CAD build for the part. Positions are in the model's coordinates, mm. A direction names the side the tool comes from. Round coordinates to 2 decimals unless told otherwise and drop trailing zeros. Loops run counter-clockwise (first coordinate to the right, second up) from the corner with the lowest first, then second, coordinate; pieces in that order, holes last.
from build123d import *

# Parameters (mm, degrees)
SKETCH_1_W          = 27.7
SKETCH_1_H          = 27.5
EXTRUDE_1_DEPTH     = 2
SKETCH_2_R          = 0.75
SKETCH_2_W          = 18
SKETCH_2_H          = 4.15
CUT_EXTRUDE_1_DEPTH = 20.61848618
SKETCH_2_3_W        = 25
SKETCH_2_3_H        = 19
CUT_EXTRUDE_2_DEPTH = 1
EXTRUDE_START       = -1
SKETCH_3_R          = 0.7
EXTRUDE_2_DEPTH     = 2


with BuildPart() as part:
    # 草图1 → 凸台-拉伸1 (new body)
    with BuildSketch(Plane.XY):
        Rectangle(SKETCH_1_W, SKETCH_1_H)
    extrude(amount=EXTRUDE_1_DEPTH)

    # 草图2 → 切除-拉伸1 (cut, through all)
    with BuildSketch(Plane.XY.offset(2)):
        with Locations((-11.7, 11.85)):
            Circle(SKETCH_2_R)
        with Locations((11.7, 11.85)):
            Circle(SKETCH_2_R)
        with Locations((-11.7, -11.85)):
            Circle(SKETCH_2_R)
        with Locations((11.7, -11.85)):
            Circle(SKETCH_2_R)
        with Locations((0, 11.675)):
            Rectangle(SKETCH_2_W, SKETCH_2_H)
    extrude(amount=-CUT_EXTRUDE_1_DEPTH, mode=Mode.SUBTRACT)

    # 草图2<3> → 切除-拉伸2 (cut)
    with BuildSketch(Plane.XY.offset(2)):
        with Locations((0, 0.1)):
            Rectangle(SKETCH_2_3_W, SKETCH_2_3_H)
    extrude(amount=-CUT_EXTRUDE_2_DEPTH, mode=Mode.SUBTRACT)

    # 草图3 → 凸台-拉伸2 (add)
    # profile 1 of 2: a face of its own
    with BuildSketch(Plane.XY.offset(1).offset(EXTRUDE_START)):
        Polygon((-17.5, -8.75), (-12.5, -8.75), (-12.5, -3.75), (-17.5, -3.75), (-17.5, -4.396520298), align=None)
        with Locations((-15.5, -5.75)):
            Circle(SKETCH_3_R, mode=Mode.SUBTRACT)
    # profile 2 of 2: a face of its own
    with BuildSketch(Plane.XY.offset(1).offset(EXTRUDE_START)):
        Polygon((12.5, -8.75), (17.5, -8.75), (17.5, -4.396520298), (17.5, -3.75), (12.5, -3.75), align=None)
        with Locations((15.5, -5.75)):
            Circle(SKETCH_3_R, mode=Mode.SUBTRACT)
    extrude(amount=EXTRUDE_2_DEPTH)


solid = part.part
Item 1: Cut at A-A (x = -15.5). List the corners of the cut face in (y, z), plus the area to 3 significant figures.
Verdict:
outline: (-8.75, 0) - (-6.45, 0) - (-6.45, 2) - (-8.75, 2) - close; (-5.05, 0) - (-3.75, 0) - (-3.75, 2) - (-5.05, 2) - close
area: 7.20 mm2
Item 2: Mould opens along Y. For faces 6 (the cylindrical face through (12.415, 12.075, 1.014)), 7 (the flat face through (0, -13.75, 1)), 8 (the flat face through (-17.5, -6, 1)) say: released by +Y, released by -Y, zero draft, split by the parting line, or undercut.
Verdict:
face 6: undercut
face 7: released by -Y
face 8: zero draft
Item 3: Cut at D-D (z = 1.55). List the corners of the cut face in (x, y), plus the area to 3 significant figures.
Verdict:
outline: (-17.5, -8.75) - (-13.85, -8.75) - (-13.85, -13.75) - (13.85, -13.75) - (13.85, -8.75) - (17.5, -8.75) - (17.5, -3.75) - (13.85, -3.75) - (13.85, 13.75) - (9, 13.75) - (9, 9.6) - (12.5, 9.6) - (12.5, -9.4) - (-12.5, -9.4) - (-12.5, 9.6) - (-9, 9.6) - (-9, 13.75) - (-13.85, 13.75) - (-13.85, -3.75) - (-17.5, -3.75) - close; hole circle Ø1.4 at (-15.5, -5.75); hole circle Ø1.5 at (-11.7, -11.85); hole circle Ø1.5 at (-11.7, 11.85); hole circle Ø1.5 at (11.7, -11.85); hole circle Ø1.5 at (11.7, 11.85); hole circle Ø1.4 at (15.5, -5.75)
area: 238 mm2
Item 4: Cut at C-C (y = 11.85). List the corners of the cut face in (x, z), plus the area to 3 significant figures.
Verdict:
outline: (-13.85, 0) - (-12.45, 0) - (-12.45, 2) - (-13.85, 2) - close; (-10.95, 0) - (-9, 0) - (-9, 2) - (-10.95, 2) - close; (9, 0) - (10.95, 0) - (10.95, 2) - (9, 2) - close; (12.45, 0) - (13.85, 0) - (13.85, 2) - (12.45, 2) - close
area: 13.4 mm2
Item 5: Wall check: L1, parallel to Y at x = 11.7, z = 0.5; L2, parallel to Y at x = -11.7, z = 1.15; L3, parallel to X at y = 9.25, z = 1.2. Give the ranges that are in metal, low to high.
Verdict:
L1: y = -13.75 to -12.6, -11.1 to 11.1, 12.6 to 13.75
L2: y = -13.75 to -12.6, -11.1 to -9.4, 9.6 to 11.1, 12.6 to 13.75
L3: x = -13.85 to -12.5, 12.5 to 13.85
Item 6: Flat gauge pins, fed straight in: P1, Ø1.1, axis at x = 3, z = 0.5, coming from the +Y side; P2, Ø1, axis at x = 15.5, z = 1, coming from the -Y side; P3, Ø1.1, axis at y = 1.5, z = 1.5, coming from the -X side. Where does each tip first touch, or does it go through?
Verdict:
P1: stops at y = 9.6
P2: stops at y = -8.75
P3: stops at x = -13.85
Item 7: Cut at B-B (y = -5.75). List the corners of the cut face in (x, z), plus the area to 3 significant figures.
Verdict:
outline: (-17.5, 0) - (-16.2, 0) - (-16.2, 2) - (-17.5, 2) - close; (-14.8, 0) - (14.8, 0) - (14.8, 2) - (12.5, 2) - (12.5, 1) - (-12.5, 1) - (-12.5, 2) - (-14.8, 2) - close; (16.2, 0) - (17.5, 0) - (17.5, 2) - (16.2, 2) - close
area: 39.4 mm2
Item 8: 3-axis set-ups, long thin cutter, end or side, ignore diameter. For faces 1 (the flat face through (-16, -3.75, 1)), 2 (the flat face through (16, -3.75, 1)), 3 (the flat face through (-0.1, 9.6, 0.5)), 4 (the flat face through (16, -8.75, 1)), 5 (the flat face through (-12.5, 0, 1.5)): which of +Z, -Z, +X, -X, +Y, -Y reach the whole face in a straight line?
Verdict:
face 1: +Z, -Z, -X, +Y
face 2: +Z, -Z, +X, +Y
face 3: +Z, -Z, +Y
face 4: +Z, -Z, +X, -Y
face 5: +Z
